Can you work these out from the model? Positions are in its coordinate system, mm. Face numbers are marked on the shaded views. A direction names the side the tool comes from. Give positions to 0.01 mm unless a question says otherwise; leave off trailing zeros. Order: outer loops, then holes, each group sorted by start corner. A loop starts at its lowest first (then second) coordinate and runs counter-clockwise, first axis right, second up. Notation, with made-up numbers: (-10, -22.75) -> (-1, -22.75) arc R19 ccw to (-1, 13.25) -> close; hole circle Ø11 at (-3.75, 86.25). An arc over 180 degrees is marked (long way). Answer as a JSON object with one key per item and string values.
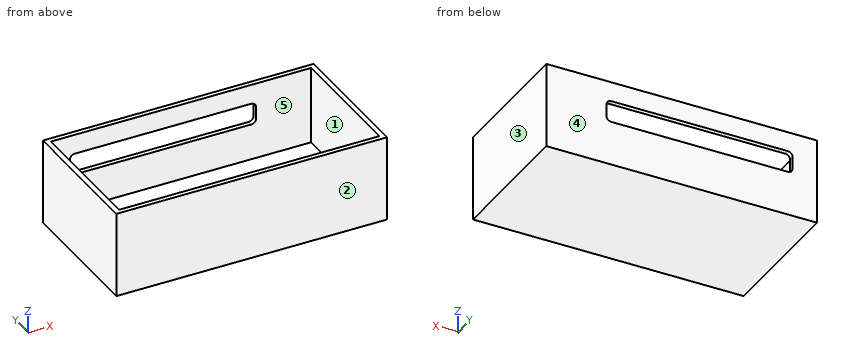
```python
from build123d import *

# Parameters (mm, degrees)
SKETCH009_W  = 111.2
SKETCH009_H  = 12.9
PAD007_DEPTH = 30
FILLET001_R  = 3
SKETCH_W     = 161.6
SKETCH_H     = 82.3
PAD_DEPTH    = 51.2
SKETCH001_W  = 155.4
SKETCH001_H  = 76.5
POCKET_DEPTH = 46.3


with BuildPart() as tubecutout:
    # Sketch009 → Pad007 (new body)
    with BuildSketch(Plane(origin=(-10.7, 54, 33), x_dir=(1, 0, 0), z_dir=(0, -1, 0))):
        Rectangle(SKETCH009_W, SKETCH009_H)
    extrude(amount=PAD007_DEPTH)

    # Fillet001
    fillet001_edges = [tubecutout.edges().sort_by_distance(p)[0] for p in [
        (-66.3, 39, 39.45),
        (-66.3, 39, 26.55),
        (44.9, 39, 39.45),
        (44.9, 39, 26.55),
    ]]
    fillet(fillet001_edges, radius=FILLET001_R)


with BuildPart() as enclosurebox:
    # Sketch → Pad (new body)
    with BuildSketch(Plane.XY):
        Rectangle(SKETCH_W, SKETCH_H)
    extrude(amount=PAD_DEPTH)

    # Sketch001 → Pocket (cut)
    with BuildSketch(Plane.XY.offset(51.2)):
        Rectangle(SKETCH001_W, SKETCH001_H)
    extrude(amount=-POCKET_DEPTH, mode=Mode.SUBTRACT)

    # Cut: cut TubeCutout
    add(tubecutout.part, mode=Mode.SUBTRACT)


solid = enclosurebox.part
```
1. If we section it at A-A on x = -7: Please give me the cut outline in (y, z).
Worked answers:
{"outline": "(-41.15, 0) -> (41.15, 0) -> (41.15, 26.55) -> (38.25, 26.55) -> (38.25, 4.9) -> (-38.25, 4.9) -> (-38.25, 51.2) -> (-41.15, 51.2) -> close; (38.25, 39.45) -> (41.15, 39.45) -> (41.15, 51.2) -> (38.25, 51.2) -> close"}
2. Will this pin go through, and if not, where does the flat tip stop? pin 1 Ø4 at (x, z) = (9, 29) entering from +Y.
Worked answers:
{"pin 1": "y = -38.25"}
3. If we mould it in two halves opening along X, with no side actions, what happens to the marked faces 3, 4 and 5? For each: +X half, -X half, draft (parallel to the pull), parting line (faces both ways), or undercut.
Worked answers:
{"face 3": "+X half", "face 4": "draft", "face 5": "undercut"}
4. If we section it at B-B on z = 22.5: Please give me the cut outline in (x, y), then the cut area to 3 significant figures.
Worked answers:
{"outline": "(-80.8, -41.15) -> (80.8, -41.15) -> (80.8, 41.15) -> (-80.8, 41.15) -> close; hole (-77.7, -38.25) -> (77.7, -38.25) -> (77.7, 38.25) -> (-77.7, 38.25) -> close", "area": "1,410 mm²"}
5. If we section it at D-D on z = 31.5: Please give me the cut outline in (x, y).
Worked answers:
{"outline": "(-80.8, -41.15) -> (80.8, -41.15) -> (80.8, 41.15) -> (44.9, 41.15) -> (44.9, 38.25) -> (77.7, 38.25) -> (77.7, -38.25) -> (-77.7, -38.25) -> (-77.7, 38.25) -> (-66.3, 38.25) -> (-66.3, 41.15) -> (-80.8, 41.15) -> close"}
6. For the marked faces 1 and 2, which set-ups out of +Z, -Z, +X, -X, +Y, -Y let a thin tool reach every point of the face, with its end or its side?
Worked answers:
{"face 1": "+Z", "face 2": "+Z, -Z, +X, -X, -Y"}
7. Please list where these lines run through material, in increasing order: L1, parallel to X at y = -32, z = 26.5; L2, parallel to Y at x = -52.5, z = 10.5; L3, parallel to Z at x = 0.5, y = 8.
Worked answers:
{"L1": "-80.8 to -77.7, 77.7 to 80.8", "L2": "-41.15 to -38.25, 38.25 to 41.15", "L3": "0 to 4.9"}
8. If we section it at C-C on y = 6: Please give me the cut outline in (x, z).
Worked answers:
{"outline": "(-80.8, 0) -> (80.8, 0) -> (80.8, 51.2) -> (77.7, 51.2) -> (77.7, 4.9) -> (-77.7, 4.9) -> (-77.7, 51.2) -> (-80.8, 51.2) -> close"}
